```python
from build123d import *

# Parameters (mm, degrees)
SKETCH1_W                               = 140
SKETCH1_H                               = 140
BASE_PLATE_DEPTH                        = 3
BASE_PLATE_CORNER_ROUNDING_R            = 5
SKETCH2_R                               = 2.5
V_WHEEL_SLOTS_AND_HOLES_DEPTH           = 4
SKETCH4_R                               = 1.5
MOTOR_MOUNT_HOLES_DEPTH                 = 4
MOTOR_MOUNT_HOLES_PATTERN_COUNT         = 2
MOTOR_MOUNT_HOLES_PATTERN_PITCH         = 31
MOTOR_MOUNT_HOLES_PATTERN_COUNT_DIR2    = 2
MOTOR_MOUNT_HOLES_PATTERN_PITCH_DIR2    = 31
SKETCH5_R                               = 12.5
MOTOR_HOLE_DEPTH                        = 4
SKETCH6_R                               = 2.5
THREADED_ROD_BLOCK_MOUNTING_HOLES_DEPTH = 4
SKETCH7_R                               = 1.5
ENDSTOP_MOUNTING_HOLES_DEPTH            = 4
WIRE_ROUTING_SLOTS_DEPTH                = 4


with BuildPart() as part:
    # Sketch1 → Base Plate (new body)
    with BuildSketch(Plane(origin=(0, 0, 0), x_dir=(0, 0, -1), z_dir=(1, 0, 0))):
        with Locations((0, 70)):
            Rectangle(SKETCH1_W, SKETCH1_H)
    extrude(amount=BASE_PLATE_DEPTH)

    # Base Plate Corner Rounding
    base_plate_corner_rounding_edges = [part.edges().sort_by_distance(p)[0] for p in [
        (1.5, 140, 70),
        (1.5, 140, -70),
        (1.5, 0, -70),
        (1.5, 0, 70),
    ]]
    fillet(base_plate_corner_rounding_edges, radius=BASE_PLATE_CORNER_ROUNDING_R)

    # Sketch2 → V Wheel Slots and Holes (cut, through all)
    with BuildSketch(Plane(origin=(3, 0, 0), x_dir=(0, 0, -1), z_dir=(1, 0, 0))):
        with Locations((60, 70)):
            Circle(SKETCH2_R)
        with Locations((-60, 70)):
            Circle(SKETCH2_R)
        with Locations((60, 10)):
            Circle(SKETCH2_R)
        with Locations((60, 130)):
            Circle(SKETCH2_R)
        with BuildLine():
            Line((-9.413957086, 14.198501159), (10.282197974, 10.725537606))
            ThreePointArc((10.282197974, 10.725537606), (12.310096913, 7.829397779), (9.413957086, 5.801498841))
            Line((9.413957086, 5.801498841), (-10.282197974, 9.274462394))
            ThreePointArc((-10.282197974, 9.274462394), (-12.310096913, 12.170602221), (-9.413957086, 14.198501159))
        make_face()
        with BuildLine():
            Line((0.725537606, 80.282197974), (4.198501159, 60.586042914))
            ThreePointArc((4.198501159, 60.586042914), (2.170602221, 57.689903087), (-0.725537606, 59.717802026))
            Line((-0.725537606, 59.717802026), (-4.198501159, 79.413957086))
            ThreePointArc((-4.198501159, 79.413957086), (-2.170602221, 82.310096913), (0.725537606, 80.282197974))
        make_face()
    extrude(amount=-V_WHEEL_SLOTS_AND_HOLES_DEPTH, mode=Mode.SUBTRACT)

    # Sketch4 → Motor Mount Holes (cut, through all)
    with BuildSketch(Plane(origin=(3, 0, 0), x_dir=(0, 0, -1), z_dir=(1, 0, 0))):
        with Locations((-64.35, 134.35)):
            Circle(SKETCH4_R)
    motor_mount_holes = extrude(amount=-MOTOR_MOUNT_HOLES_DEPTH, mode=Mode.SUBTRACT)

    # Motor Mount Holes Pattern: Motor Mount Holes 2 × 2
    with Locations(*[(0, -j * MOTOR_MOUNT_HOLES_PATTERN_PITCH_DIR2, -i * MOTOR_MOUNT_HOLES_PATTERN_PITCH) for i in range(MOTOR_MOUNT_HOLES_PATTERN_COUNT) for j in range(MOTOR_MOUNT_HOLES_PATTERN_COUNT_DIR2) if (i, j) != (0, 0)]):
        add(motor_mount_holes, mode=Mode.SUBTRACT)

    # Sketch5 → Motor Hole (cut, through all)
    with BuildSketch(Plane(origin=(3, 0, 0), x_dir=(0, 0, -1), z_dir=(1, 0, 0))):
        with Locations((-48.85, 118.85)):
            Circle(SKETCH5_R)
    extrude(amount=-MOTOR_HOLE_DEPTH, mode=Mode.SUBTRACT)

    # Sketch6 → Threaded Rod Block Mounting Holes (cut, through all)
    with BuildSketch(Plane(origin=(3, 0, 0), x_dir=(0, 0, -1), z_dir=(1, 0, 0))):
        with Locations((-8, 30)):
            Circle(SKETCH6_R)
        with Locations((-28, 30)):
            Circle(SKETCH6_R)
    extrude(amount=-THREADED_ROD_BLOCK_MOUNTING_HOLES_DEPTH, mode=Mode.SUBTRACT)

    # Sketch7 → Endstop Mounting Holes (cut, through all)
    with BuildSketch(Plane(origin=(3, 0, 0), x_dir=(0, 0, -1), z_dir=(1, 0, 0))):
        with Locations((-62.5, 51)):
            Circle(SKETCH7_R)
        with Locations((-62.5, 40)):
            Circle(SKETCH7_R)
        with Locations((62.5, 51)):
            Circle(SKETCH7_R)
        with Locations((62.5, 40)):
            Circle(SKETCH7_R)
        with Locations((40, 132.5)):
            Circle(SKETCH7_R)
        with Locations((29, 132.5)):
            Circle(SKETCH7_R)
        with Locations((40, 7.5)):
            Circle(SKETCH7_R)
        with Locations((29, 7.5)):
            Circle(SKETCH7_R)
    extrude(amount=-ENDSTOP_MOUNTING_HOLES_DEPTH, mode=Mode.SUBTRACT)

    # Sketch8 → Wire Routing Slots (cut, through all)
    with BuildSketch(Plane(origin=(3, 0, 0), x_dir=(0, 0, -1), z_dir=(1, 0, 0))):
        with BuildLine():
            Line((65, 105), (65, 95))
            ThreePointArc((65, 95), (60, 90), (55, 95))
            Line((55, 95), (55, 105))
            ThreePointArc((55, 105), (60, 110), (65, 105))
        make_face()
        with BuildLine():
            Line((-35, 85), (-35, 75))
            ThreePointArc((-35, 75), (-40, 70), (-45, 75))
            Line((-45, 75), (-45, 85))
            ThreePointArc((-45, 85), (-40, 90), (-35, 85))
        make_face()
        with BuildLine():
            Line((-55, 15), (-45, 15))
            ThreePointArc((-45, 15), (-40, 10), (-45, 5))
            Line((-45, 5), (-55, 5))
            ThreePointArc((-55, 5), (-60, 10), (-55, 15))
        make_face()
    extrude(amount=-WIRE_ROUTING_SLOTS_DEPTH, mode=Mode.SUBTRACT)


solid = part.part
```
CAD build for the part. Positions are in the model's coordinates, mm. A direction names the side the tool comes from. Round coordinates to 2 decimals unless told otherwise and drop trailing zeros. Write each loop counter-clockwise with the first axis right and the second up, starting at its lowest first coordinate (ties: lowest second). Pieces come first, ordered by that corner, then holes. Notation, with made-up numbers: (27.25, 78) - (78.25, 78) arc R14 ccw to (78.25, 97) - close; hole circle Ø7 at (3, 30.5). An arc over 180 degrees is marked (long way). Return JSON: item names as keys, results as strings. Group by question number.
Item 1: Band-saw the part on B-B on x = 2.5. State how many separate pieces and enclosed holes the cut face has, plus the area to 3 significant figures.
Item 2: Band-saw the part on A-A on z = 28. List the corners of the cut face in (x, y), plus the area to 3 significant figures.
Item 3: Flat gauge pin, fed straight in: pin 1 Ø4 at (y, z) = (53, -26.5) entering from -X. Where does the tip first touch, or does it go through?
Item 4: Probe probe 1 along Y at (x, z) = (2.3, -60); probe 2 along Y at (x, z) = (1.95, -40); probe 3 along Y at (x, z) = (1.6, -59). List the from-to ranges inside material, lowest first.
Item 5: Mould opens along Y. For faces 3 (the face through (2, 100, -55)), 4 (the face through (1, 0, 1)), 5 (the face through (3, 71, 17)), 6 (the face through (2, 138, -69)) say: +Y half, -Y half, draft (parallel to the pull), parting line (faces both ways), or undercut.
Item 6: 3-axis set-ups, long thin cutter, end or side, ignore diameter. For faces 1 (the face through (2, 5, 50)), 2 (the face through (2, 2, 69)): which of +Z, -Z, +X, -X, +Y, -Y reach the whole face in a straight line?
Resolved:
{
 "1": {"separate pieces": "1", "enclosed holes": "24", "area": "18,100 mm²"},
 "2": {"outline": "(0, 0) - (3, 0) - (3, 27.5) - (0, 27.5) - close; (0, 32.5) - (3, 32.5) - (3, 140) - (0, 140) - close", "area": "405 mm²"},
 "3": {"pin 1": "stops at x = 0"},
 "4": {"probe 1": "y = 0 to 7.5, 12.5 to 67.5, 72.5 to 90, 110 to 127.5, 132.5 to 140", "probe 2": "y = 0 to 6, 9 to 131, 134 to 140", "probe 3": "y = 0 to 7.71, 12.29 to 67.71, 72.29 to 90.1, 109.9 to 127.71, 132.29 to 140"},
 "5": {"face 3": "undercut", "face 4": "-Y half", "face 5": "draft", "face 6": "+Y half"},
 "6": {"face 1": "+X, -X", "face 2": "+Z, +X, -X, -Y"}
}
